```python
from build123d import *

# Parameters (mm, degrees)
SKETCH2_R           = 3.5814
BOSS_EXTRUDE1_DEPTH = 5.08
SKETCH3_R           = 3.5814
CUT_EXTRUDE1_DEPTH  = 5.08


# Read off the part's stored shape, not the designer's step: Shell3
with BuildPart() as part:
    # Sketch1 → Revolve1 (revolve)
    with BuildSketch(Plane.XY):
        Polygon((0, 0), (-33.401, 0), (-19.138871581, 228.6), (0, 228.6), align=None)
    revolve(axis=Axis((0, 228.6, 0), (0, -1, 0)))

    # Sketch2 → Boss-Extrude1 (add)
    with BuildSketch(Plane(origin=(0, 228.6, 0), x_dir=(1, 0, 0), z_dir=(0, 1, 0))):
        with Locations(Location((0, 0, 0), (0, 0, 180))):
            Circle(SKETCH2_R)
    extrude(amount=BOSS_EXTRUDE1_DEPTH)

    # Sketch3 → Cut-Extrude1 (cut)
    with BuildSketch(Plane.XZ):
        with Locations(Location((0, 0, 0), (0, 0, 180))):
            Circle(SKETCH3_R)
    extrude(amount=-CUT_EXTRUDE1_DEPTH, mode=Mode.SUBTRACT)

    # Shell3 outline → Shell3 (revolve, cut)
    with BuildSketch(Plane.XY):
        Polygon((6.1214, 7.62), (6.1214, 2.54), (30.697593373, 2.54), (16.752401141, 226.06), (1.0414, 226.06), (1.0414, 231.14), (0, 231.14), (0, 7.62), align=None)
    revolve(axis=Axis((0, 0, 0), (0, 1, 0)), mode=Mode.SUBTRACT)


solid = part.part
```
Model file for the job. Use its own axes, mm. A direction names the side the tool comes from. Give positions to 0.01 mm unless a question says otherwise; leave off trailing zeros. Write each loop counter-clockwise with the first axis right and the second up, starting at its lowest first coordinate (ties: lowest second). Pieces come first, ordered by that corner, then holes. Notation, with made-up numbers: M -1,-38 L 17,-38 A30 ccw 17,-2 Z; hole C 2.5,-19 d4. An arc over 180 degrees is marked long. Use a Markdown table: item, result.
1) Pull direction Y, two halves, no side cores. Call faces 1 (the conical face through (5.67, 115.9, 25.55)), 2 (the flat face through (0, 0, 7)), 3 (the flat face through (-6.4, 2.54, -0.4)), 4 (the cylindrical face through (-1.65, 2.5, 3.18)): +Y half, -Y half, draft (parallel to the pull), parting line (faces both ways), or undercut.
Responses:
| item | result |
|---|---|
| face 1 | +Y half |
| face 2 | -Y half |
| face 3 | undercut |
| face 4 | draft |
2) Cut at B-B (y = 116.5). List the corners of the cut face in (x, z), and give its area (3 significant figures).
Responses:
| item | result |
|---|---|
| outline | C 0,0 d52.27; hole C 0,0 d47.18 |
| area | 398 mm2 |
3) Tool access for faces 5 (the flat face through (0, 233.68, 0)), 6 (the cylindrical face through (-1.327, 5.044, 5.976)), 7 (the cylindrical face through (-1.65, 231.1, -3.18)), 8 (the flat face through (0, 5.08, 0)): list every direction of +Z, -Z, +X, -X, +Y, -Y with a clear straight run to the whole face (end or side of a thin tool).
Responses:
| item | result |
|---|---|
| face 5 | +Z, -Z, +X, -X, +Y |
| face 6 | none |
| face 7 | +Y |
| face 8 | -Y |
4) Pin check, flat tips, straight feed: pin 1 (1.7 mm diameter, centred on x = 0, z = 0, fed in from -Y); pin 2 (1.5 mm diameter, centred on x = 16, z = 0, fed in from +Y); pin 3 (1.5 mm diameter, centred on x = -1.5, y = 131.5, fed in from +Z). Stop position of each tip, or through.
Responses:
| item | result |
|---|---|
| pin 1 | stops at y = 5.08 |
| pin 2 | stops at y = 228.6 |
| pin 3 | stops at z = 25.21 |
5) Cut at A-A (y = 145.5). List the corners of the cut face in (x, z), and give its area (3 significant figures).
Responses:
| item | result |
|---|---|
| outline | C 0,0 d48.65; hole C 0,0 d43.56 |
| area | 369 mm2 |
6) Drill centre lines: line 1 (Z direction, x = 0, y = 3.1); line 2 (Z direction, x = 0, y = 3.4); line 3 (X direction, y = 181, z = 14). Where is each one in solid material? Low to high. Write a range as from..to.
Responses:
| item | result |
|---|---|
| line 1 | z = -33.21..-30.66, -6.12..-3.58, 3.58..6.12, 30.66..33.21 |
| line 2 | z = -33.19..-30.64, -6.12..-3.58, 3.58..6.12, 30.64..33.19 |
| line 3 | x = -17.11..-13.67, 13.67..17.11 |
